Source: CAD feature listing. Evaluate the final solid. Frame: model axes, mm. A direction names the side the tool comes from. Round coordinates to 2 decimals unless told otherwise and drop trailing zeros. Loops run counter-clockwise (first coordinate to the right, second up) from the corner with the lowest first, then second, coordinate; pieces in that order, holes last.
Item 1: First-contact query: P1, Ø4, axis at x = -7.95, y = 7.95, coming from the +Z side; P2, Ø5, axis at x = 7.5, z = -8.5, coming from the -Y side. Flat tips, straight axial feed; report the tip coordinate or a pass-through.
Item 2: Section query B-B on x = -11.5. Return loops of the section in (y, z).
Item 3: Section query A-A on z = -6.5. Return loops of the section in (x, y), then the cut area to 3 significant figures.
Item 4: Access query for faces 1 (the cylindrical face through (7.478, 5.807, -0.986)), 2 (the cylindrical face through (-8.51, -9.02, -6.06)). Directions: +Z, -Z, +X, -X, +Y, -Y. A direction counts if a zero-diameter tool reaches every point of the face in a straight line with its end or side. Return the directions, or none.
Item 5: Pull-direction query (Y, two-part tool) for faces 3 (the cylindrical face through (-8.6, 8.967, -6.056)), 4 (the cylindrical face through (0.24, 16.25, -4.93)), 5 (the flat face through (-14, 0, -5)), 6 (the cylindrical face through (8.111, 9.145, -6.056)); classes: released by +Y, released by -Y, zero draft, split by the parting line, or undercut.
Item 6: Section query C-C on y = 12. Return loops of the section in (x, z), then the cut area to 3 significant figures.
Item 7: Ray query, L1, parallel to X at y = -8.5, z = -3.75; L2, parallel to X at y = -8, z = -0.75; L3, parallel to Y at x = 7.75, z = -9.25. Return the intervals inside material, ascending.
```python
from build123d import *

# Parameters (mm, degrees)
SKETCH1_R                      = 16.25
BOSS_EXTRUDE1_DEPTH            = 10
CUT_EXTRUDE1_DEPTH             = 26.06242207
CUT_EXTRUDE1_DEPTH_BACK        = 26.06242207
SKETCH2_W                      = 10
SKETCH2_H                      = 16.5
CBORE_FOR_M2_SHCS1_D           = 2.4
CBORE_FOR_M2_SHCS1_CBORE_D     = 4.4
CBORE_FOR_M2_SHCS1_CBORE_DEPTH = 2


with BuildPart() as part:
    # Sketch1 → Boss-Extrude1 (new body)
    with BuildSketch(Plane.XY):
        Circle(SKETCH1_R)
    extrude(amount=-BOSS_EXTRUDE1_DEPTH)

    # Sketch2 → Cut-Extrude1 (cut, two sides: drawn at the far end of the back side and taken through both)
    with BuildSketch(Plane.XY.offset(-CUT_EXTRUDE1_DEPTH_BACK)):
        with Locations((19, 0)):
            Rectangle(SKETCH2_W, SKETCH2_H)
        with Locations((-19, 0)):
            Rectangle(SKETCH2_W, SKETCH2_H)
    extrude(amount=CUT_EXTRUDE1_DEPTH + CUT_EXTRUDE1_DEPTH_BACK, mode=Mode.SUBTRACT)

    # CBORE for M2 SHCS1 (through all)
    with Locations(Plane.XY):
        with Locations((-7.954951288, 7.954951288), (7.954951288, 7.954951288), (7.954951288, -7.954951288), (-7.954951288, -7.954951288)):
            CounterBoreHole(CBORE_FOR_M2_SHCS1_D / 2, CBORE_FOR_M2_SHCS1_CBORE_D / 2, CBORE_FOR_M2_SHCS1_CBORE_DEPTH)


solid = part.part
```
Data:
1. P1: stops at z = -2
1. P2: stops at y = -15.46
2. outline: (-11.48, -10) - (11.48, -10) - (11.48, 0) - (-11.48, 0) - close
3. outline: (-14, -8.25) arc R16.25 ccw to (14, -8.25) - (14, 8.25) arc R16.25 ccw to (-14, 8.25) - close; hole circle Ø2.4 at (-7.95, -7.95); hole circle Ø2.4 at (-7.95, 7.95); hole circle Ø2.4 at (7.95, -7.95); hole circle Ø2.4 at (7.95, 7.95)
3. area: 761 mm2
4. face 1: +Z
4. face 2: +Z, -Z
5. face 3: undercut
5. face 4: released by +Y
5. face 5: zero draft
5. face 6: undercut
6. outline: (-10.96, -10) - (10.96, -10) - (10.96, 0) - (-10.96, 0) - close
6. area: 219 mm2
7. L1: x = -13.85 to -9.02, -6.89 to 6.89, 9.02 to 13.85
7. L2: x = -14 to -10.15, -5.76 to 5.76, 10.15 to 14
7. L3: y = -14.28 to -9.14, -6.77 to 6.77, 9.14 to 14.28
